from build123d import *
from build123d.topology import SkipClean

# Parameters (mm, degrees)
EXTRUDE_1_DEPTH      = 80
SKETCH_2_R           = 1.7
CUT_EXTRUDE_1_DEPTH  = 100
SKETCH_3_R           = 1.7
CUT_EXTRUDE_2_DEPTH  = 100
SKETCH_4_R           = 3.4
CUT_EXTRUDE_3_DEPTH  = 26.5
SKETCH_5_R           = 3.4
CUT_EXTRUDE_4_DEPTH  = 13
EXTRUDE_START        = 3
EXTRUDE_2_DEPTH      = 3
EXTRUDE_3_DEPTH      = 9.5
EXTRUDE_4_DEPTH      = 7
SKETCH_14_R          = 1.5
CUT_EXTRUDE_6_DEPTH  = 14
SKETCH_18_W          = 14
SKETCH_18_H          = 3
CUT_EXTRUDE_9_DEPTH  = 20
SKETCH_19_R          = 3
CUT_EXTRUDE_10_DEPTH = 3
FILLET_4_R           = 1
CHAMFER_2_SIZE       = 2
SKETCH_20_R          = 6
CUT_EXTRUDE_11_DEPTH = 15
SKETCH_23_W          = 5.624944444
SKETCH_23_H          = 15.463858562
CUT_EXTRUDE_14_DEPTH = 30
SKETCH_25_W          = 14
SKETCH_25_H          = 41.8
CUT_EXTRUDE_16_DEPTH = 5
FILLET_6_R           = 4
EXTRUDE_START_2      = 2
EXTRUDE_5_DEPTH      = 2
EXTRUDE_6_DEPTH      = 2


# Some blends are built 0.0001 mm under size
with BuildPart() as part:
    # 草图1 → 凸台-拉伸1 (new body)
    with BuildSketch(Plane(origin=(0, 0, 0), x_dir=(1, 0, 0), z_dir=(0, 1, 0))):
        with BuildLine():
            Line((-15, 0), (-30, 0))
            ThreePointArc((-30, 0), (0, -30), (30, 0))
            Line((30, 0), (15, 0))
            Line((15, 0), (15, -15.2))
            Line((15, -15.2), (-15, -15.2))
            Line((-15, -15.2), (-15, 0))
        make_face()
    extrude(amount=EXTRUDE_1_DEPTH)

    # 草图2 → 切除-拉伸1 (cut)
    with BuildSketch(Plane.XY):
        with Locations(Location((-10, 37, 0), (0, 0, 180))):
            Circle(SKETCH_2_R)
        with Locations(Location((-10, 67, 0), (0, 0, 180))):
            Circle(SKETCH_2_R)
        with Locations(Location((10, 37, 0), (0, 0, 180))):
            Circle(SKETCH_2_R)
        with Locations(Location((10, 67, 0), (0, 0, 180))):
            Circle(SKETCH_2_R)
    extrude(amount=CUT_EXTRUDE_1_DEPTH, mode=Mode.SUBTRACT)

    # 草图3 → 切除-拉伸2 (cut)
    with BuildSketch(Plane(origin=(0, 0, 0), x_dir=(-1, 0, 0), z_dir=(0, 0, -1))):
        with Locations((23.5, 65)):
            Circle(SKETCH_3_R)
        with Locations((-23.5, 65)):
            Circle(SKETCH_3_R)
        with Locations((23.5, 15)):
            Circle(SKETCH_3_R)
        with Locations((-23.5, 15)):
            Circle(SKETCH_3_R)
    extrude(amount=-CUT_EXTRUDE_2_DEPTH, mode=Mode.SUBTRACT)

    # 草图4 → 切除-拉伸3 (cut)
    with BuildSketch(Plane(origin=(0, 0, 40), x_dir=(-1, 0, 0), z_dir=(0, 0, -1))):
        with Locations((-23.5, 65)):
            Circle(SKETCH_4_R)
        with Locations((-23.5, 15)):
            Circle(SKETCH_4_R)
        with Locations((23.5, 65)):
            Circle(SKETCH_4_R)
        with Locations((23.5, 15)):
            Circle(SKETCH_4_R)
    extrude(amount=CUT_EXTRUDE_3_DEPTH, mode=Mode.SUBTRACT)

    # 草图5 → 切除-拉伸4 (cut)
    with BuildSketch(Plane(origin=(0, 0, 40), x_dir=(-1, 0, 0), z_dir=(0, 0, -1))):
        with Locations((-10, 37)):
            Circle(SKETCH_5_R)
        with Locations((10, 37)):
            Circle(SKETCH_5_R)
        with Locations((10, 67)):
            Circle(SKETCH_5_R)
        with Locations((-10, 67)):
            Circle(SKETCH_5_R)
    extrude(amount=CUT_EXTRUDE_4_DEPTH, mode=Mode.SUBTRACT)

    # 草图6 → 凸台-拉伸2 (add)
    with SkipClean():  # the faces are left unmerged after this step: merging them gives an invalid solid
        with BuildSketch(Plane.XZ.offset(EXTRUDE_START)):
            with BuildLine():
                Line((-30, 0), (30, 0))
                ThreePointArc((30, 0), (0, 30), (-30, 0))
            make_face()
        extrude(amount=-EXTRUDE_2_DEPTH)

    # 草图7 → 凸台-拉伸3 (add)
    with SkipClean():  # the faces are left unmerged after this step: merging them gives an invalid solid
        with BuildSketch(Plane.XZ.offset(3)):
            with BuildLine():
                Line((-6, 0), (6, 0))
                ThreePointArc((6, 0), (0, 6), (-6, 0))
            make_face()
        extrude(amount=EXTRUDE_3_DEPTH)

    # 草图13 → 凸台-拉伸4 (add, symmetric)
    with SkipClean():  # the faces are left unmerged after this step: merging them gives an invalid solid
        with BuildSketch(Plane(origin=(0, 0, 0), x_dir=(0, 0, -1), z_dir=(1, 0, 0))):
            with BuildLine():
                Line((-15.2, 100), (-60, 100))
                add(Edge.make_bspline(
                    [(-60, 100), (-54.458111129, 76.859605584), (-30, 70)],
                    knots=[0, 0, 0, 1, 1, 1], degree=2))
                Line((-30, 70), (-15.2, 70))
                Line((-15.2, 70), (-15.2, 100))
            make_face()
        extrude(amount=EXTRUDE_4_DEPTH, both=True)

    # 草图14 → 切除-拉伸6 (cut)
    with SkipClean():  # the faces are left unmerged after this step: merging them gives an invalid solid
        with BuildSketch(Plane.ZY.offset(7)):
            with Locations((32, 90)):
                Circle(SKETCH_14_R)
            with Locations((52, 90)):
                Circle(SKETCH_14_R)
        extrude(amount=-CUT_EXTRUDE_6_DEPTH, mode=Mode.SUBTRACT)

    # 草图18 → 切除-拉伸9 (cut)
    with SkipClean():  # the faces are left unmerged after this step: merging them gives an invalid solid
        with BuildSketch(Plane(origin=(0, 100, 0), x_dir=(1, 0, 0), z_dir=(0, 1, 0))):
            with Locations((0, -16.7)):
                Rectangle(SKETCH_18_W, SKETCH_18_H)
        extrude(amount=-CUT_EXTRUDE_9_DEPTH, mode=Mode.SUBTRACT)

    # 草图19 → 切除-拉伸10 (cut)
    with SkipClean():  # the faces are left unmerged after this step: merging them gives an invalid solid
        with BuildSketch(Plane(origin=(0, 0, 0), x_dir=(1, 0, 0), z_dir=(0, 1, 0))):
            Circle(SKETCH_19_R)
        extrude(amount=-CUT_EXTRUDE_10_DEPTH, mode=Mode.SUBTRACT)

    # 圆角4
    # the kernel refuses this fillet: 1 mm, written as the material it adds along each edge
    with BuildSketch(Plane(origin=(0, -3, 0), x_dir=(-1, 0, 0), z_dir=(0, 0, -1))) as fillet_4_piece_1:
        with BuildLine():
            CenterArc((3 - FILLET_4_R, FILLET_4_R), FILLET_4_R, 270, 90)
            Line((3 - FILLET_4_R, 0), (3, 0))
            Line((3, 0), (3, FILLET_4_R))
        make_face()
    revolve(axis=Axis((0, -3, 0), (0, 1, 0)), revolution_arc=180)

    # 倒角2
    chamfer_2_edges = [part.edges().sort_by_distance(p)[0] for p in [
        (0, 0, 3),
    ]]
    chamfer(chamfer_2_edges, length=CHAMFER_2_SIZE - 0.0001)  # a hair under: the kernel refuses the full size

    # 草图20 → 切除-拉伸11 (cut)
    with BuildSketch(Plane.XZ.offset(3)):
        with Locations(Location((0, 20.5, 0), (0, 0, 270))):
            Circle(SKETCH_20_R)
    extrude(amount=-CUT_EXTRUDE_11_DEPTH, mode=Mode.SUBTRACT)

    # 草图23 → 切除-拉伸14 (cut)
    with BuildSketch(Plane(origin=(0, 0, 15.2), x_dir=(-1, 0, 0), z_dir=(0, 0, -1))):
        with Locations((0, 4.268070719)):
            Rectangle(SKETCH_23_W, SKETCH_23_H)
    extrude(amount=-CUT_EXTRUDE_14_DEPTH, mode=Mode.SUBTRACT)

    # 草图25 → 切除-拉伸16 (cut)
    with BuildSketch(Plane(origin=(0, 100, 0), x_dir=(1, 0, 0), z_dir=(0, 1, 0))):
        with Locations((0, -39.1)):
            Rectangle(SKETCH_25_W, SKETCH_25_H)
    extrude(amount=-CUT_EXTRUDE_16_DEPTH, mode=Mode.SUBTRACT)

    # 圆角6
    fillet_6_edges = [part.edges().sort_by_distance(p)[0] for p in [
        (3.4999997, 95, 58.513859135),
    ]]
    fillet(fillet_6_edges, radius=FILLET_6_R)

    # 草图26 → 凸台-拉伸5 (add)
    with BuildSketch(Plane.XZ.offset(3).offset(EXTRUDE_START_2)):
        with BuildLine():
            ThreePointArc((30, 0), (22.185289796, 20.194378343), (2.812472222, 29.86787572))
            Line((2.812472222, 29.86787572), (2.812472222, 25.8))
            ThreePointArc((2.812472222, 25.8), (0, 14.5), (-2.812472222, 25.8))
            Line((-2.812472222, 25.8), (-2.812472222, 29.86787572))
            ThreePointArc((-2.812472222, 29.86787572), (-22.185289796, 20.194378343), (-30, 0))
            Line((-30, 0), (-6, 0))
            ThreePointArc((-6, 0), (0, 6), (6, 0))
            Line((6, 0), (30, 0))
        make_face()
    extrude(amount=-EXTRUDE_5_DEPTH)

    # 草图27 → 凸台-拉伸6 (add)
    with BuildSketch(Plane.XZ.offset(12.5)):
        with BuildLine():
            Line((-6, 0), (6, 0))
            ThreePointArc((6, 0), (0, 6), (-6, 0))
        make_face()
    extrude(amount=EXTRUDE_6_DEPTH)


solid = part.part
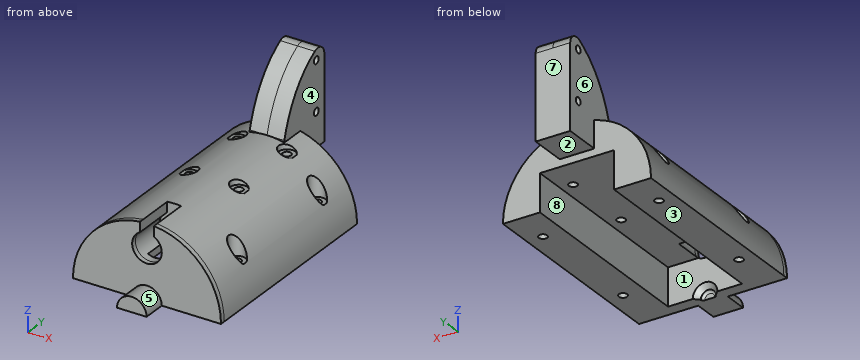
The model under review builds one solid part; all positions refer to its coordinate system, in mm. Face numbers are marked on the shaded views. A direction names the side the tool comes from. Round coordinates to 2 decimals unless told otherwise and drop trailing zeros. Write each loop counter-clockwise with the first axis right and the second up, starting at its lowest first coordinate (ties: lowest second). Pieces come first, ordered by that corner, then holes. Notation, with made-up numbers: M -27,-27.5 L 5,-27.5 A15 cw 5,-19.5 Z; hole C 66,-39 d5. An arc over 180 degrees is marked long. Answer as CSV lines item,"result". Start each with the question number.
Q1. The part is to be moulded in two halves that separate along X. For the marked faces 5, 6, 7 and 8, say which applies: +X half, -X half, draft (parallel to the pull), parting line (faces both ways), or undercut.
Q2. Consider section A-A, the plane y = 37. Give the boundary of the cut face in (x, z) (3 decimals), then the cut area to 3 significant figures.
Q3. Consider section B-B, the plane y = 4. Give the boundary of the cut face in (x, z).
Q4. Wall thickness on line 1 along Y through (x, z) = (10, 22.25); line 2 along Z through (x, y) = (1, 90); line 3 along X through (y, z) = (65, 5.25): over which ranges is each line inside the solid? List them lowest first.
Q5. Clearance check with flat-ended pins moving along their axes: P1, Ø1.9, axis at x = 10.5, y = 37.5, coming from the +Z side; P2, Ø0.9, axis at x = -4.5, z = 29.5, coming from the -Y side; P3, Ø7, axis at x = -10.5, y = 67, coming from the +Z side; P4, Ø10, axis at x = -23.5, z = 12, coming from the +Y side. State where each tip first meets the part, or that it passes through.
Q6. Consider section D-D, the plane z = 11. Give the boundary of the cut face in (x, y).
Q7. Consider section C-C, the plane x = 23.5. Give the boundary of the cut face in (y, z), then the cut area to 3 significant figures.
Q8. Tool access review of the marked faces 1, 2, 3 and 4: name each direction out of +Z, -Z, +X, -X, +Y, -Y from which nothing blocks a thin tool from reaching the whole face with its end or side.
Result set:
1,face 5,"parting line"
1,face 6,"-X half"
1,face 7,"draft"
1,face 8,"undercut"
2,outline,"M -30,0 L -15,0 L -15,15.2 L -11.7,15.2 L -11.7,27 L -13.077,27 A30 ccw Z; M -8.3,15.2 L 8.3,15.2 L 8.3,27 L 6.6,27 L 6.6,29.265 A30 ccw -6.6,29.265 L -6.6,27 L -8.3,27 Z; M 11.7,15.2 L 15,15.2 L 15,0 L 30,0 A30 ccw 13.077,27 L 11.7,27 Z"
2,area,"861 mm²"
3,outline,"M -30,0 L -15,0 L -15,15.2 L -2.81,15.2 A6 cw -2.81,25.8 L -2.81,29.87 A30 ccw Z; M 2.81,15.2 L 15,15.2 L 15,0 L 30,0 A30 ccw 2.81,29.87 L 2.81,25.8 A6 cw Z"
4,line 1,"y = -5 to 35.3, 38.7 to 65.3, 68.7 to 80"
4,line 2,"z = 18.2 to 30.5, 33.5 to 50.5, 53.5 to 56.21"
4,line 3,"x = -29.54 to -25.2, -21.8 to -15, 15 to 21.8, 25.2 to 29.54"
5,P1,"passes through"
5,P2,"stops at y = -5"
5,P3,"stops at z = 28.44"
5,P4,"stops at y = 80"
6,outline,"M -27.91,-5 L 27.91,-5 L 27.91,80 L 15,80 L 15,0 L -15,0 L -15,80 L -27.91,80 Z; hole C -23.5,15 d3.4; hole C -23.5,65 d3.4; hole C 23.5,15 d3.4; hole C 23.5,65 d3.4"
7,outline,"M -5,0 L 13.3,0 L 13.3,13.5 L 11.6,13.5 L 11.6,18.65 L -5,18.65 Z; M 16.7,0 L 63.3,0 L 63.3,13.5 L 61.6,13.5 L 61.6,18.65 L 18.4,18.65 L 18.4,13.5 L 16.7,13.5 Z; M 66.7,0 L 80,0 L 80,18.65 L 68.4,18.65 L 68.4,13.5 L 66.7,13.5 Z"
7,area,"1,420 mm²"
8,face 1,"-Z, +Y"
8,face 2,"-Z, +X, -X, +Y"
8,face 3,"-Z, +X, -X, +Y, -Y"
8,face 4,"+Z, +X, +Y"
